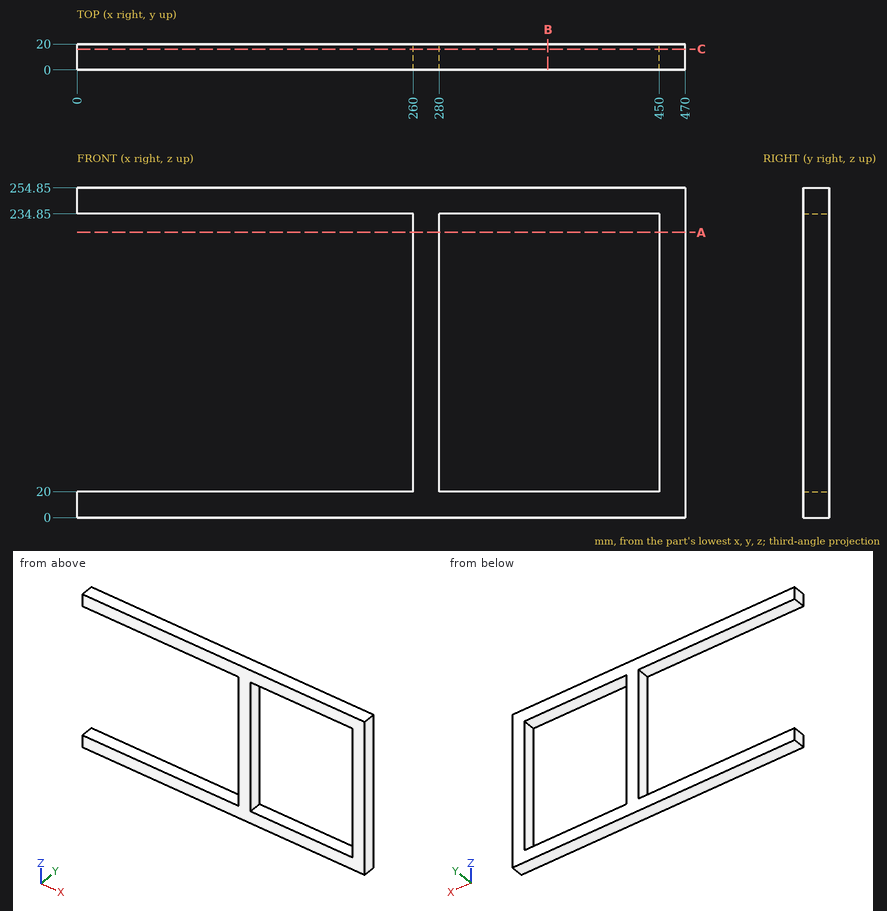
For this review, use the dimensioned drawing (mm, ordinates from the lowest corner) and the shaded views. Coordinates: 2 decimals unless noted, no trailing zeros. Loops run counter-clockwise (first coordinate to the right, second up) from the corner with the lowest first, then second, coordinate; pieces in that order, holes last. Notation, with made-up numbers: (80.5, 45) -> (91.5, 45) arc R11 ccw to (91.5, 62) -> close; hole circle Ø1 at (38, -10). An arc over 180 degrees is marked (long way). Return JSON: item names as keys, results as strings. Group by question number.
(1) Consider section C-C, the plane y = 16. Give the boundary of the cut face in (x, z), plus the area to 3 significant figures.
(2) To check wall thickness, follow L1, parallel to Z at x = 151.5, y = 2; L2, parallel to X at y = 16.75, z = 143.5. State the ranges of each line that lie inside material, in increasing order.
(3) Consider section B-B, the plane x = 364. Give the boundary of the cut face in (y, z), plus the area to 3 significant figures.
(4) Consider section A-A, the plane z = 220.5. Give the boundary of the cut face in (x, y).
(5) For pin 1 Ø1.5 at (y, z) = (15, 131.5) entering from -X, flat-tipped, find the tip position at first contact; note if it passes through.
Results below:
{
 "1": {"outline": "(0, 0) -> (470, 0) -> (470, 254.85) -> (0, 254.85) -> (0, 234.85) -> (260, 234.85) -> (260, 20) -> (0, 20) -> close; hole (280, 20) -> (450, 20) -> (450, 234.85) -> (280, 234.85) -> close", "area": "27,400 mm2"},
 "2": {"L1": "z = 0 to 20, 234.85 to 254.85", "L2": "x = 260 to 280, 450 to 470"},
 "3": {"outline": "(0, 0) -> (20, 0) -> (20, 20) -> (0, 20) -> close; (0, 234.85) -> (20, 234.85) -> (20, 254.85) -> (0, 254.85) -> close", "area": "800 mm2"},
 "4": {"outline": "(260, 0) -> (280, 0) -> (280, 20) -> (260, 20) -> close; (450, 0) -> (470, 0) -> (470, 20) -> (450, 20) -> close"},
 "5": {"pin 1": "stops at x = 260"}
}
